Autodesk Inventor part; units mm, degrees
ref_plane "YZ Plane" through (0, 0, 0) normal (1, 0, 0) x (0, 1, 0)
ref_plane "XZ Plane" through (0, 0, 0) normal (0, 1, 0) x (-1, 0, 0)
ref_plane "XY Plane" through (0, 0, 0) normal (0, 0, 1) x (1, 0, 0)
sketch "Sketch1" plane through (0, 0, 0) normal (0, 0, 1) x (1, 0, 0)
  line L0 (20.25, 10) -> (-20.25, 10)
  line L1 (-20.25, 10) -> (-20.25, -10)
  line L2 (-20.25, -10) -> (20.25, -10)
  line L3 (20.25, -10) -> (20.25, 10)
  line L4 (20.25, 10) -> (-20.25, -10) construction
  line L5 (-20.25, 10) -> (20.25, -10) construction
  line L6 (-27, 10) -> (-27, 6.25)
  line L7 (27, -10) -> (27, -6.25)
  line L8 (27, 10) -> (-27, -10) construction
  line L9 (-27, 10) -> (27, -10) construction
  line L10 (20.25, -10) -> (27, -10)
  line L11 (20.25, 10) -> (27, 10)
  line L12 (-20.25, 10) -> (-27, 10)
  line L13 (-20.25, -10) -> (-27, -10)
  line L14 (24.25, 5) -> (-24.25, 5) construction
  line L15 (-24.25, 5) -> (-24.25, -5) construction
  line L16 (-24.25, -5) -> (24.25, -5) construction
  line L17 (24.25, -5) -> (24.25, 5) construction
  line L18 (24.25, 5) -> (-24.25, -5) construction
  line L19 (-24.25, 5) -> (24.25, -5) construction
  circle A0 centre (-24.25, 5) radius 1
  line L20 (-20.25, 0) -> (20.25, 0) construction
  line L21 (0, 10) -> (0, -10) construction
  circle A1 centre (-24.25, -5) radius 1
  circle A2 centre (24.25, 5) radius 1
  circle A3 centre (24.25, -5) radius 1
  line L22 (-27, 3.75) -> (-27, -3.75)
  line L23 (-27, 6.25) -> (-27, 3.75)
  line L24 (-27, -6.25) -> (-27, -10)
  line L25 (-27, -3.75) -> (-27, -6.25)
  line L26 (27, -3.75) -> (27, 3.75)
  line L27 (27, -6.25) -> (27, -3.75)
  line L28 (27, 3.75) -> (27, 6.25)
  line L29 (27, 6.25) -> (27, 10)
  line L30 (-22.25, -10) -> (-22.25, 10)
  line L31 (22.25, -10) -> (22.25, 10)
  line L32 (-27, 10) -> (-27, 12)
  line L33 (-27, 12) -> (27, 12)
  line L34 (27, 12) -> (27, 10)
  point P0 (0, 0)
  point P1 (0, 0)
  point P2 (0, 0)
  dimension "d0" = 40.5
  dimension "d1" = 20
  dimension "d2" = 54
  dimension "d3" = 48.5
  dimension "d4" = 10
  dimension "d6" = 2
  dimension "d7" = 2
  dimension "d8" = 2
  dimension "d9" = 2
extrude "Extrusion1" add sketch "Sketch1" along normal blind 3 contours L11 L31 L10 L3 | L0 L12 L32 L33 L34 L11 | L1 L13 L30 L12 | L11 L29 L28 L26 L27 L7 L10 L31 | L30 L13 L24 L25 L22 L23 L6 L12
extrude "Extrusion2" add sketch "Sketch1" against normal blind 9 contours L11 L31 L10 L3 | L0 L12 L32 L33 L34 L11 | L1 L13 L30 L12
extrude "Extrusion3" add sketch "Sketch1" against normal blind 25 contours L11 L31 L10 L3 | L0 L12 L32 L33 L34 L11
sketch "Sketch2" plane through (0, 0, -25) normal (0, 0, -1) x (-1, 0, 0)
  line L0 (27, 10) -> (27, 12)
  line L1 (27, 12) -> (-27, 12)
  line L2 (-27, 12) -> (-27, 10)
  line L3 (-22.25, -10) -> (-20.25, -10)
  line L4 (-32, -10) -> (32, -10)
  line L5 (32, -10) -> (32, 32)
  line L6 (32, 32) -> (-32, 32)
  line L7 (-32, 32) -> (-32, -10)
  point P0 (0, 0)
  dimension "d16" = 20
  dimension "d17" = 5
  dimension "d18" = 5
extrude "Extrusion4" add sketch "Sketch2" along normal blind 4
sketch "Sketch3" plane through (0, 0, -9) normal (0, 0, -1) x (-1, 0, 0)
  line L0 (22.25, 10) -> (20.25, 10)
  line L1 (20.25, 10) -> (20.25, -10)
  line L2 (22.25, -10) -> (22.25, 10)
  line L3 (20.25, 4.4217) -> (22.25, 4.4217)
  point P0 (0, 0)
extrude "Extrusion5" add sketch "Sketch3" along normal up to next
properties part number "podstawa"
Work out the finished part from the listing and answer in its coordinate system (mm). A direction names the side the tool comes from. Round coordinates to 2 decimals unless told otherwise and drop trailing zeros. Write each loop counter-clockwise with the first axis right and the second up, starting at its lowest first coordinate (ties: lowest second). Pieces come first, ordered by that corner, then holes. Notation, with made-up numbers: (-24.5, 64) - (16.5, 64) arc R25 ccw to (16.5, 84) - close; hole circle Ø7 at (2, -4.5). An arc over 180 degrees is marked (long way). Return JSON: item names as keys, results as strings. Group by question number.
Q1. For faces 1 (the flat face through (20.25, 0, -11)), 2 (the flat face through (25, 0, 0)), 3 (the flat face through (0, 12, -11)), 4 (the flat face through (-25, 0, 0)), determine the directions among +Z, -Z, +X, -X, +Y, -Y from which every point of the face is accessible in a straight line to the end or side of a thin tool.
Q2. Find the intervals of material crossed by L1, parallel to Y at x = -24.25, z = 1.1; L2, parallel to Z at x = -13.5, y = 29.5; L3, parallel to Y at x = 22, z = -6.5, in increasing order.
Q3. The part is cut by section C-C on z = -20. Write down the section's boundary in (x, y), then the cut area to 3 significant figures.
Q4. Each of these flat-tipped pins is pushed along its axis until it touches: pin 1 Ø6.5 at (y, z) = (-1.5, -7) entering from +X; pin 2 Ø10 at (y, z) = (-1.5, -10.5) entering from -X; pin 3 Ø12 at (x, z) = (-3.5, -9.5) entering from -Y. Where does it stop, or does it pass through?
Q5. The mould has two halves that part along Y. Classify faces 5 (the flat face through (-20.25, 2, -8)), 6 (the flat face through (25, 10, -12)), 7 (the cylindrical face through (-24.987, -5.676, 1.479)), 8 (the cylindrical face through (23.513, 4.324, 1.479)): released by +Y, released by -Y, zero draft, split by the parting line, or undercut.
Q6. The part is cut by section D-D on x = 24.25. Write down the section's boundary in (y, z).
Q7. The part is cut by section B-B on x = 11. Write down the section's boundary in (y, z).
Q8. The part is cut by section A-A on y = -5. Write down the section's boundary in (x, z), then the cut area to 4 significant figures.
Solved:
{
 "1": {"face 1": "+Z, -Y", "face 2": "+X, -Y", "face 3": "+Z, +X, -X, +Y", "face 4": "-X, -Y"},
 "2": {"L1": "-10 to -6, -4 to 4, 6 to 12", "L2": "-29 to -25", "L3": "-10 to 12"},
 "3": {"outline": "(-27, 10) - (-22.25, 10) - (-22.25, 4.42) - (-20.25, 4.42) - (-20.25, 10) - (20.25, 10) - (20.25, -10) - (22.25, -10) - (22.25, 10) - (27, 10) - (27, 12) - (-27, 12) - close", "area": "159 mm²"},
 "4": {"pin 1": "x = 22.25", "pin 2": "x = -22.25", "pin 3": "y = 10"},
 "5": {"face 5": "zero draft", "face 6": "released by -Y", "face 7": "undercut", "face 8": "undercut"},
 "6": {"outline": "(-10, -29) - (32, -29) - (32, -25) - (12, -25) - (12, 3) - (6, 3) - (6, 0) - (10, 0) - (10, -25) - (-10, -25) - close; (-10, 0) - (-6, 0) - (-6, 3) - (-10, 3) - close; (-4, 0) - (4, 0) - (4, 3) - (-4, 3) - close"},
 "7": {"outline": "(-10, -29) - (32, -29) - (32, -25) - (12, -25) - (12, 3) - (10, 3) - (10, -25) - (-10, -25) - close"},
 "8": {"outline": "(-32, -29) - (32, -29) - (32, -25) - (22.25, -25) - (22.25, 0) - (23.25, 0) - (23.25, 3) - (20.25, 3) - (20.25, -25) - (-32, -25) - close; (-27, 0) - (-25.25, 0) - (-25.25, 3) - (-27, 3) - close; (-23.25, 0) - (-22.25, 0) - (-22.25, -9) - (-20.25, -9) - (-20.25, 3) - (-23.25, 3) - close; (25.25, 0) - (27, 0) - (27, 3) - (25.25, 3) - close", "area": "352.5 mm²"}
}
